Read the model definition and answer for the solid it produces. Units are mm, in the model's axes. Face numbers are marked on the shaded views. Coordinates: 2 decimals unless noted, no trailing zeros. Loops run counter-clockwise (first coordinate to the right, second up) from the corner with the lowest first, then second, coordinate; pieces in that order, holes last. Notation, with made-up numbers: (32, 29.25) -> (45, 29.25) arc R25 cw to (45, 48.25) -> close; hole circle Ø4 at (78.25, -33). An arc over 180 degrees is marked (long way). Answer as a JSON object with one key per item and string values. Group by question number.
Q1. The part is cut by section C-C on y = -10. Write down the section's boundary in (x, z), and give its area (3 significant figures).
Q2. Straight lines are drawn through the part: line 1 along Y through (x, z) = (0, 58); line 2 along X through (y, z) = (7.5, 73); line 3 along Y through (x, z) = (22, 72.5). For each, find the intervals that lie inside material, in ascending order. Write a range as [from, to].
Q3. The part is cut by section B-B on z = 11.5. Write down the section's boundary in (x, y), and give its area (3 significant figures).
Q4. Each of these flat-tipped pins is pushed along its axis until it touches: P1, Ø6, axis at x = -31, y = -34.5, coming from the -Z side; P2, Ø2, axis at x = 3, z = 73, coming from the +Y side; P3, Ø1, axis at y = -31, z = 80.5, coming from the -X side (3 decimals); P4, Ø3, axis at x = -24.5, y = -34, coming from the +Z side. Where does it stop, or does it pass through?
Q5. Determine the mould class of the marked faces 1, 2 and 3 for opening direction Y: released by +Y, released by -Y, zero draft, split by the parting line, or undercut.
Q6. The part is cut by section A-A on y = 0. Write down the section's boundary in (x, z).
Autodesk Inventor part; units mm, degrees
ref_plane "YZ Plane" through (0, 0, 0) normal (1, 0, 0) x (0, 1, 0)
ref_plane "XZ Plane" through (0, 0, 0) normal (0, 1, 0) x (-1, 0, 0)
ref_plane "XY Plane" through (0, 0, 0) normal (0, 0, 1) x (1, 0, 0)
sketch "Sketch1" plane through (0, 0, 0) normal (0, 0, 1) x (1, 0, 0)
  circle A0 centre (0, 0) radius 50
  circle A1 centre (0, 0) radius 25
  dimension "d0" = 100
  dimension "d1" = 50
extrude "Extrusion1" add sketch "Sketch1" along normal blind 100
sketch "Sketch2" plane through (0, 0, 100) normal (0, 0, 1) x (1, 0, 0)
  circle A0 centre (0, 0) radius 50
  line L0 (0, 50) -> (43.3013, 25)
  line L1 (43.3013, 25) -> (43.3013, -25)
  line L2 (43.3013, -25) -> (0, -50)
  line L3 (0, -50) -> (-43.3013, -25)
  line L4 (-43.3013, -25) -> (-43.3013, 25)
  line L5 (-43.3013, 25) -> (0, 50)
  circle A1 centre (0, 0) radius 50
  dimension "d4" = 0
extrude "Extrusion2" cut sketch "Sketch2" against normal blind 100 contours A0 L1 | L0 A0 | A0 L2 | L5 A0 | A0 L3 | L4 A0
fillet "Fillet1" radius 2 12 edges at (0, 50, 50) (21.6506, 37.5, 100) (-21.6506, 37.5, 100) (43.3013, 25, 50) (43.3013, -25, 50) (43.3013, 0, 100) (-43.3013, 25, 50) (-43.3013, 0, 100) (-43.3013, -25, 50) (-21.6506, -37.5, 100) (0, -50, 50) (21.6506, -37.5, 100)
fillet "Fillet2" radius 2 12 edges at (0, 49.6906, 0) (21.6506, 37.5, 0) (43.0333, 24.8453, 0) (43.3013, 0, 0) (43.0333, -24.8453, 0) (21.6506, -37.5, 0) (0, -49.6906, 0) (-21.6506, -37.5, 0) (-43.0333, -24.8453, 0) (-43.3013, 0, 0) (-43.0333, 24.8453, 0) (-21.6506, 37.5, 0)
properties part number "Nut" material "Iron, Malleable"
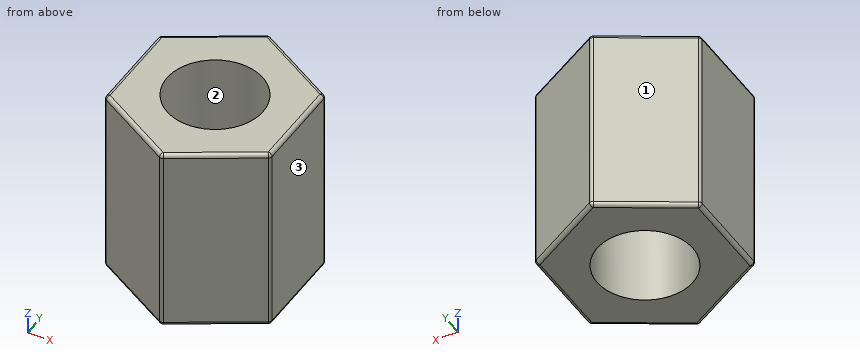
Final values:
{
 "1": {"outline": "(-43.3, 2) arc R2 ccw to (-41.3, 0) -> (-22.91, 0) -> (-22.91, 100) -> (-41.3, 100) arc R2 ccw to (-43.3, 98) -> close; (22.91, 0) -> (41.3, 0) arc R2 ccw to (43.3, 2) -> (43.3, 98) arc R2 ccw to (41.3, 100) -> (22.91, 100) -> close", "area": "4,070 mm2"},
 "2": {"line 1": "y = [-49.69, -25], [25, 49.69]", "line 2": "x = [-43.3, -23.85], [23.85, 43.3]", "line 3": "y = [-37.3, -11.87], [11.87, 37.3]"},
 "3": {"outline": "(-43.3, -23.85) arc R2 ccw to (-42.3, -25.58) -> (-1, -49.42) arc R2 ccw to (1, -49.42) -> (42.3, -25.58) arc R2 ccw to (43.3, -23.85) -> (43.3, 23.85) arc R2 ccw to (42.3, 25.58) -> (1, 49.42) arc R2 ccw to (-1, 49.42) -> (-42.3, 25.58) arc R2 ccw to (-43.3, 23.85) -> close; hole circle Ø50 at (0, 0)", "area": "4,530 mm2"},
 "4": {"P1": "stops at z = 0.31", "P2": "stops at y = 48.85", "P3": "stops at x = -33.775", "P4": "stops at z = 100"},
 "5": {"face 1": "released by +Y", "face 2": "undercut", "face 3": "zero draft"},
 "6": {"outline": "(-43.3, 2) arc R2 ccw to (-41.3, 0) -> (-25, 0) -> (-25, 100) -> (-41.3, 100) arc R2 ccw to (-43.3, 98) -> close; (25, 0) -> (41.3, 0) arc R2 ccw to (43.3, 2) -> (43.3, 98) arc R2 ccw to (41.3, 100) -> (25, 100) -> close"}
}
